The figure shows three views and two pictorial views of one solid part (mm, origin at its lowest corner). Answer the questions. Coordinates: 2 decimals unless noted, no trailing zeros. Order: outer loops, then holes, each group sorted by start corner. A loop starts at its lowest first (then second) coordinate and runs counter-clockwise, first axis right, second up. Notation, with made-up numbers: (-37.75, -22) -> (4.25, -22) arc R13 ccw to (4.25, 1) -> close; hole circle Ø7 at (-29.75, 54). An arc over 180 degrees is marked (long way). Write item = value, one per line. Start each with the question number.
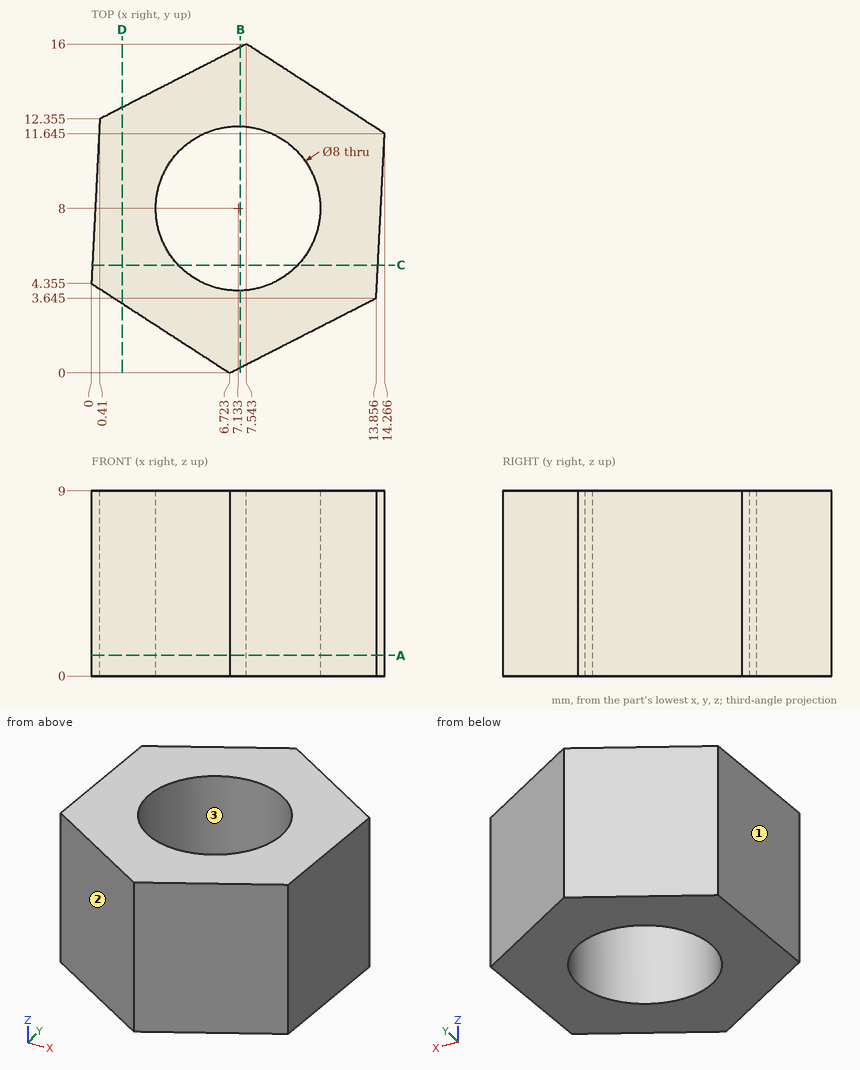
Item 1: Consider probe 1 along X at (y, z) = (6.75, 0.5) (1 decimal); probe 2 along Y at (x, z) = (7, 3); probe 3 along X at (y, z) = (11.5, 6.5) (1 decimal). Determine where each line is inside the solid, lowest interval first.
Item 2: For a pull along Y with two mould halves and no side action, classify the marked faces 1, 2 and 3 as pulls with the +Y half, pulls with the -Y half, needs draft (parallel to the pull), parting line crosses it, or undercut.
Item 3: Section B-B, the plane x = 7.25 is taken. Give the vertices of the cut face in (y, z).
Item 4: Each of these flat-tipped pins is pushed along its axis until it touches: pin 1 (5 mm diameter, centred on y = 2, z = 5, fed in from +X); pin 2 (1 mm diameter, centred on y = 12, z = 4.5, fed in from -X); pin 3 (3 mm diameter, centred on x = 5.5, y = 7.5, fed in from -Z); pin 4 (1.5 mm diameter, centred on x = 12.5, z = 7, fed in from -Y). Where does it stop, or does it pass through?
Item 5: Section A-A, the plane z = 1 is taken. Give the vertices of the cut face in (x, y) (1 decimal).
Item 6: Section D-D, the plane x = 1.5 is taken. Give the vertices of the cut face in (y, z).
Item 7: Section C-C, the plane y = 5.25 is taken. Give the vertices of the cut face in (x, z).
A:
q1.probe_1 = 0.1 to 3.3, 10.9 to 14
q1.probe_2 = 0.14 to 4, 12 to 15.72
q1.probe_3 = 0.4 to 5.2, 9.1 to 14.3
q2.face_1 = pulls with the +Y half
q2.face_2 = pulls with the -Y half
q2.face_3 = undercut
q3.outline = (0.27, 0) -> (4, 0) -> (4, 9) -> (0.27, 9) -> close; (12, 0) -> (15.85, 0) -> (15.85, 9) -> (12, 9) -> close
q4.pin_1 = 13.9
q4.pin_2 = 0.37
q4.pin_3 = through
q4.pin_4 = 2.57
q5.outline = (0, 4.4) -> (6.7, 0) -> (13.9, 3.6) -> (14.3, 11.6) -> (7.5, 16) -> (0.4, 12.4) -> close; hole circle Ø8 at (7.1, 8)
q6.outline = (3.38, 0) -> (12.91, 0) -> (12.91, 9) -> (3.38, 9) -> close
q7.outline = (0.05, 0) -> (4.23, 0) -> (4.23, 9) -> (0.05, 9) -> close; (10.04, 0) -> (13.94, 0) -> (13.94, 9) -> (10.04, 9) -> close
